The listing builds one solid part. Answer for the finished solid, in the listing's coordinates (mm). A direction names the side the tool comes from. Give positions to 0.01 mm unless a question says otherwise; leave off trailing zeros. Write each loop counter-clockwise with the first axis right and the second up, starting at its lowest first coordinate (ties: lowest second). Pieces come first, ordered by that corner, then holes.
```python
from build123d import *

# Parameters (mm, degrees)
SKETCH1_R               = 2.5
BOSS_EXTRUDE1_DEPTH     = 23
CHAMFER1_SIZE           = 0.5
CUT_EXTRUDE1_DEPTH      = 24.270152556
CUT_EXTRUDE1_DEPTH_BACK = 24.270152556
SKETCH2_W               = 0.5
SKETCH2_H               = 18


with BuildPart() as part:
    # Sketch1 → Boss-Extrude1 (new body)
    with BuildSketch(Plane(origin=(0, 0, 0), x_dir=(1, 0, 0), z_dir=(0, 1, 0))):
        with Locations(Location((0, 0, 0), (0, 0, 270))):
            Circle(SKETCH1_R)
    extrude(amount=BOSS_EXTRUDE1_DEPTH)

    # Chamfer1
    chamfer1_edges = [part.edges().sort_by_distance(p)[0] for p in [
        (0, 23, -2.5),
    ]]
    chamfer(chamfer1_edges, length=CHAMFER1_SIZE)

    # Sketch2 → Cut-Extrude1 (cut, two sides: drawn at the far end of the back side and taken through both)
    with BuildSketch(Plane(origin=(0, 0, 0), x_dir=(0, 0, -1), z_dir=(1, 0, 0)).offset(-CUT_EXTRUDE1_DEPTH_BACK)):
        with Locations((2.25, 14)):
            Rectangle(SKETCH2_W, SKETCH2_H)
    extrude(amount=CUT_EXTRUDE1_DEPTH + CUT_EXTRUDE1_DEPTH_BACK, mode=Mode.SUBTRACT)


solid = part.part
```
Item 1: Consider probe 1 along X at (y, z) = (7.75, -0.1); probe 2 along Z at (x, y) = (-0.05, 20); probe 3 along X at (y, z) = (6, -1.7). Determine where each line is inside the solid, lowest interval first.
Conclusion:
probe 1: x = -2.5 to 2.5
probe 2: z = -2 to 2.5
probe 3: x = -1.83 to 1.83
Item 2: A cutting plane is placed at B-B, the plane y = 2. Give the vertices of the cut face in (x, z).
Conclusion:
outline: circle Ø5 at (0, 0)
Item 3: A cutting plane is placed at A-A, the plane y = 21.25. Give the vertices of the cut face in (x, z), plus the area to 3 significant figures.
Conclusion:
outline: (-1.5, -2) - (1.5, -2) arc R2.5 ccw (long way) to start
area: 18.6 mm2
Item 4: Which of the six approach directions +Z, -Z, +X, -X, +Y, -Y give full straight-line access (tool end or side, diameter ignored) to faces 1 (the face through (0, 14, -2)), 2 (the face through (0, 0, 0))?
Conclusion:
face 1: -Z, +X, -X, +Y
face 2: +Z, -Z, +X, -X, -Y
Item 5: Each of these flat-tipped pins is pushed along its axis until it touches: P1, Ø2.5, axis at x = 0.5, y = 15, coming from the -Z side; P2, Ø1, axis at x = -1.5, y = 4, coming from the +Z side; P3, Ø1, axis at x = 2, y = 6, coming from the +Z side. Where does it stop, or does it pass through?
Conclusion:
P1: stops at z = -2
P2: stops at z = 2.29
P3: stops at z = 2
